Geometry: see drawing. Coordinates: mm, zero at the bounding-box minimum. A direction names the side the tool comes from. Give positions to 0.01 mm unless a question says otherwise; leave off trailing zeros. Write each loop counter-clockwise with the first axis right and the second up, starting at its lowest first coordinate (ties: lowest second). Pieces come first, ordered by that corner, then holes. Notation, with made-up numbers: (-20, 56) -> (21, 56) arc R31 cw to (21, 94) -> close; hole circle Ø10 at (45.25, -29.75). An arc over 180 degrees is marked (long way). Answer as a JSON object with one key per item and string values. Group by question number.
Item 1: First-contact query: pin 1 Ø9.5 at (x, z) = (12.5, 13.5) entering from +Y; pin 2 Ø5 at (x, z) = (52, 10) entering from -Y; pin 3 Ø8.5 at (y, z) = (14.5, 14.5) entering from -X. Flat tips, straight axial feed; report the tip coordinate or a pass-through.
Item 2: Section query D-D on x = 125. Return the cut outline in (y, z).
Item 3: Access query for the marked faces 4, 5, 6, 7 and 8. Directions: +Z, -Z, +X, -X, +Y, -Y. A direction counts if a zero-diameter tool reaches every point of the face in a straight line with its end or side. Return the directions, or none.
Item 4: Section query B-B on x = 150. Return the cut outline in (y, z).
Item 5: Section query C-C on z = 35.5. Return the cut outline in (x, y).
Item 6: Pull-direction query (X, two-part tool) for the marked faces 1, 2 and 3; classes: pulls with the +X half, pulls with the -X half, needs draft (parallel to the pull), parting line crosses it, or undercut.
Item 7: Section query A-A on y = 12.5. Return the cut outline in (x, z).
Item 8: Ray query, probe 1 along Z at (x, y) = (150, 1.1); probe 2 along X at (y, z) = (8.75, 31); probe 3 along X at (y, z) = (1.6, 31). Return the intervals inside material, ascending. Write a range as from..to.
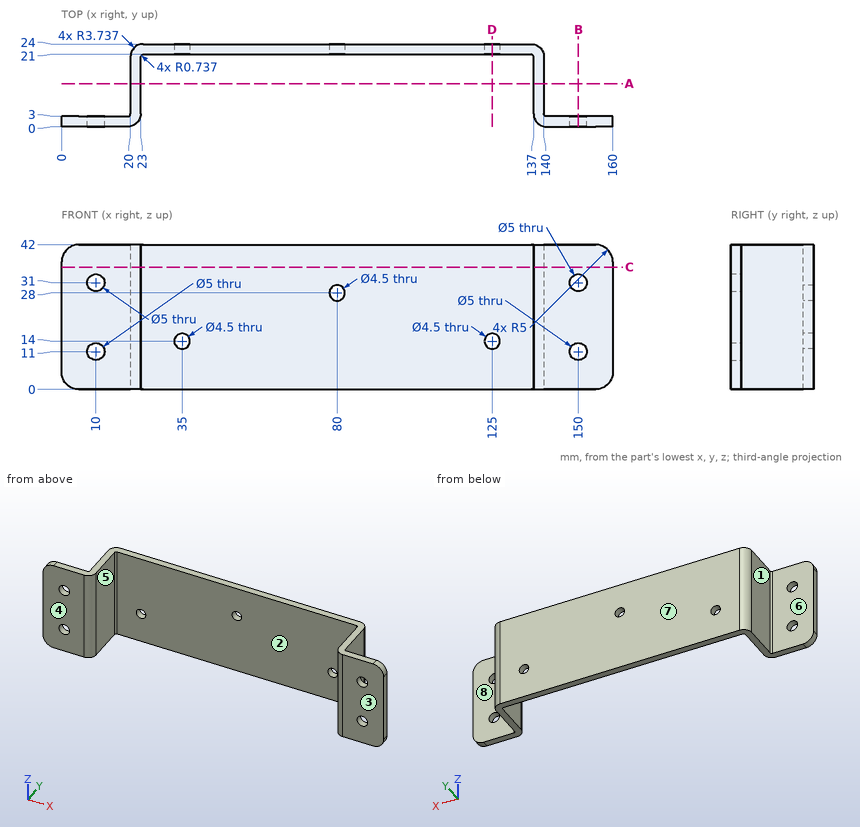
Worked answers:
{
 "1": {"pin 1": "y = 3", "pin 2": "y = 21", "pin 3": "x = 20"},
 "2": {"outline": "(21, 0) -> (24, 0) -> (24, 11.75) -> (21, 11.75) -> close; (21, 16.25) -> (24, 16.25) -> (24, 42) -> (21, 42) -> close"},
 "3": {"face 4": "+Z, -Z, +X, -X, -Y", "face 5": "+Z, -Z, -Y", "face 6": "+Z, -Z, -X, +Y", "face 7": "+Z, -Z, +X, -X, +Y", "face 8": "+Z, -Z, +X, +Y"},
 "4": {"outline": "(0, 0) -> (3, 0) -> (3, 8.5) -> (0, 8.5) -> close; (0, 13.5) -> (3, 13.5) -> (3, 28.5) -> (0, 28.5) -> close; (0, 33.5) -> (3, 33.5) -> (3, 42) -> (0, 42) -> close"},
 "5": {"outline": "(0, 0) -> (19.26, 0) arc R3.74 ccw to (23, 3.74) -> (23, 20.26) arc R0.74 cw to (23.74, 21) -> (136.26, 21) arc R0.74 cw to (137, 20.26) -> (137, 3.74) arc R3.74 ccw to (140.74, 0) -> (160, 0) -> (160, 3) -> (140.74, 3) arc R0.74 cw to (140, 3.74) -> (140, 20.26) arc R3.74 ccw to (136.26, 24) -> (23.74, 24) arc R3.74 ccw to (20, 20.26) -> (20, 3.74) arc R0.74 cw to (19.26, 3) -> (0, 3) -> close"},
 "6": {"face 1": "pulls with the -X half", "face 2": "undercut", "face 3": "needs draft"},
 "7": {"outline": "(20, 0) -> (23, 0) -> (23, 42) -> (20, 42) -> close; (137, 0) -> (140, 0) -> (140, 42) -> (137, 42) -> close"},
 "8": {"probe 1": "0..8.5, 13.5..28.5, 33.5..42", "probe 2": "20..23, 137..140", "probe 3": "0..7.5, 12.5..22.33, 137.67..147.5, 152.5..160"}
}
